Could you check a few things on this model? Use its own coordinates, in mm. A direction names the side the tool comes from. Coordinates: 2 decimals unless noted, no trailing zeros. Order: outer loops, then holes, each group sorted by start corner. A loop starts at its lowest first (then second) coordinate and runs counter-clockwise, first axis right, second up. Notation, with made-up numbers: (-13.75, 54.5) - (-2.75, 54.5) arc R18 cw to (-2.75, 89.5) - close; hole circle Ø1 at (17.25, 16.5). An arc over 180 degrees is marked (long way). One line per item, written item: value. Start each with the question number.
from build123d import *

# Parameters (mm, degrees)
SKETCH1_R           = 11.43
BOSS_EXTRUDE1_DEPTH = 6.731
BOSS_EXTRUDE2_START = -22.86
BOSS_EXTRUDE2_DEPTH = 22.86


with BuildPart() as part:
    # Sketch1 → Boss-Extrude1 (new body)
    # profile 1 of 2: a face of its own
    with BuildSketch(Plane(origin=(0, 0, 0), x_dir=(1, 0, 0), z_dir=(0, 1, 0))):
        with Locations(Location((0, 0, 0), (0, 0, 270))):
            Circle(SKETCH1_R)
        Polygon((-6.35, 0), (-3.175, -5.499261314), (3.175, -5.499261314), (6.35, 0), (3.175, 5.499261314), (-3.175, 5.499261314), align=None, mode=Mode.SUBTRACT)
    # profile 2 of 2: a face of its own
    with BuildSketch(Plane(origin=(0, 0, 0), x_dir=(1, 0, 0), z_dir=(0, 1, 0))):
        Polygon((-3.175, 5.499261314), (-6.35, 0), (-3.175, -5.499261314), (3.175, -5.499261314), (6.35, 0), (3.175, 5.499261314), align=None)
        with BuildLine():
            ThreePointArc((2.014584776, 1.499860387), (-2.51159969, 0), (2.014584776, -1.499860387))
            Line((2.014584776, -1.499860387), (2.014584776, 1.499860387))
        make_face(mode=Mode.SUBTRACT)
    extrude(amount=BOSS_EXTRUDE1_DEPTH)

    # Sketch1_3 → Boss-Extrude2 (add)
    with BuildSketch(Plane(origin=(0, 0, 0), x_dir=(1, 0, 0), z_dir=(0, 1, 0)).offset(BOSS_EXTRUDE2_START)):
        Polygon((-3.175, 5.499261314), (-6.35, 0), (-3.175, -5.499261314), (3.175, -5.499261314), (6.35, 0), (3.175, 5.499261314), align=None)
        with BuildLine():
            ThreePointArc((2.014584776, 1.499860387), (-2.51159969, 0), (2.014584776, -1.499860387))
            Line((2.014584776, -1.499860387), (2.014584776, 1.499860387))
        make_face(mode=Mode.SUBTRACT)
    extrude(amount=BOSS_EXTRUDE2_DEPTH)


solid = part.part
Q1. I want a section at D-D on x = 5.5. Please give me the cut outline in (y, z), then the cut area to 3 significant figures.
Q2. I'm going to push flat-ended pins straight in: pin 1 (3.5 mm diameter, centred on y = -7, z = 0.5, fed in from -X); pin 2 (10 mm diameter, centred on x = 8, z = -2.5, fed in from -Y); pin 3 (1.9 mm diameter, centred on x = 0, y = -16, fed in from -Z); pin 4 (1 mm diameter, centred on x = -3, y = -15.5, fed in from +Z). Where does each tip first touch, or does it pass through?
Q3. If I drill on L1, parallel to X at y = 0.5, z = 0; L2, parallel to X at y = -10.5, z = 0; L3, parallel to Z at x = 0, y = -6, over which ranges is the centre line in solid material (lowest first)?
Q4. Which directions (+Z, -Z, +X, -X, +Y, -Y) give clear straight access to the entire face, cutting with the end or side of a thin tool? Please do faces 5 (the flat face through (5, 0, -3)), 6 (the flat face through (4.785, -11.59, -2.711)), 7 (the flat face through (0, -12, -5.499)), 8 (the flat face through (-4.74, -11.59, -2.79)).
Q5. I want a section at B-B on y = -20.5. Please give me the cut outline in (x, z) (3 decimals), then the cut area to 3 significant figures.
Q6. We'd pull the mould along X, two halves only. Please class faces 1 (the flat face through (4.74, -11.59, 2.79)), 2 (the flat face through (-4.785, -11.59, 2.711)), 3 (the flat face through (2.015, -8, 0)), 4 (the cylindrical face through (-2.51, -8.27, -0.09)): +X half, -X half, draft (parallel to the pull), parting line (faces both ways), or undercut.
Q7. I want a section at A-A on x = 0. Please give me the cut outline in (y, z).
Q8. I want a section at C-C on z = -5. Please give me the cut outline in (x, y).
Values follow:
1. outline: (-22.86, -1.47) - (0, -1.47) - (0, -10.02) - (6.73, -10.02) - (6.73, 10.02) - (0, 10.02) - (0, 1.47) - (-22.86, 1.47) - close
1. area: 202 mm^2
2. pin 1: stops at x = -6.35
2. pin 2: stops at y = -22.86
2. pin 3: stops at z = -5.5
2. pin 4: stops at z = 5.5
3. L1: x = -11.43 to -2.51, 2.01 to 11.43
3. L2: x = -6.35 to -2.51, 2.01 to 6.35
3. L3: z = -5.5 to -2.51, 2.51 to 5.5
4. face 5: -Y
4. face 6: -Z, +X, -Y
4. face 7: -Z, +X, -X, -Y
4. face 8: -Z, -X, -Y
5. outline: (-6.35, 0) - (-3.175, -5.499) - (3.175, -5.499) - (6.35, 0) - (3.175, 5.499) - (-3.175, 5.499) - close; hole (2.015, -1.5) - (2.015, 1.5) arc R2.512 ccw (long way) to start
5. area: 86.0 mm^2
6. face 1: +X half
6. face 2: -X half
6. face 3: undercut
6. face 4: undercut
7. outline: (-22.86, -5.5) - (0, -5.5) - (0, -11.43) - (6.73, -11.43) - (6.73, -2.51) - (-22.86, -2.51) - close; (-22.86, 2.51) - (6.73, 2.51) - (6.73, 11.43) - (0, 11.43) - (0, 5.5) - (-22.86, 5.5) - close
8. outline: (-10.28, 0) - (-3.46, 0) - (-3.46, -22.86) - (3.46, -22.86) - (3.46, 0) - (10.28, 0) - (10.28, 6.73) - (-10.28, 6.73) - close
